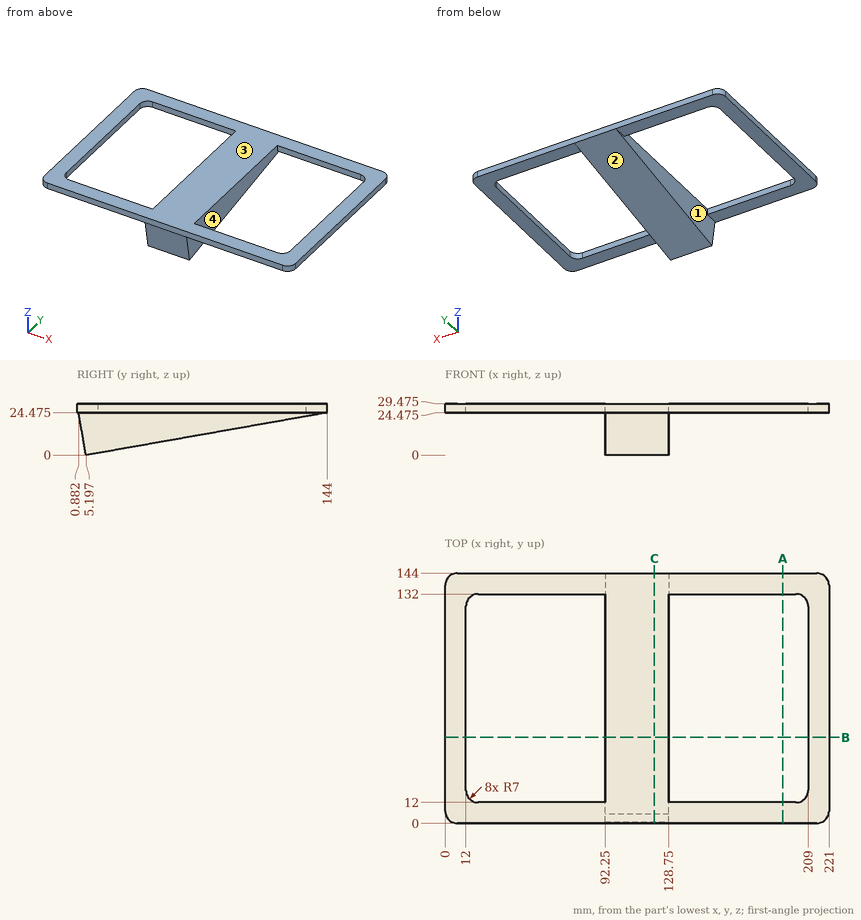
Part print with two shaded views. Sizes in mm from the minimum x, y, z corner. A direction names the side the tool comes from. Give positions to 0.01 mm unless a question says otherwise; leave off trailing zeros. Order: outer loops, then holes, each group sorted by start corner. A loop starts at its lowest first (then second) coordinate and runs counter-clockwise, first axis right, second up. Notation, with made-up numbers: M 59.5,35.25 L 114.5,35.25 A26 ccw 114.5,69.25 Z; hole C 73.25,40 d10. An arc over 180 degrees is marked long. Write item = value, one per line.
Q1. Two-plate mould, pull along X, no slides. Class the marked faces 3 and 4: pulls with the +X half, pulls with the -X half, needs draft (parallel to the pull), parting line crosses it, or undercut.
Derived:
face_3 = needs draft
face_4 = undercut
Q2. Cut at C-C, the plane x = 120.5. List the corners of the cut face in (y, z) (1 decimal), then the cut area to 3 significant figures.
Derived:
outline = M 0,24.5 L 0.9,24.5 L 5.2,0 L 144,24.5 L 144,29.5 L 0,29.5 Z
area = 2,470 mm2
Q3. Drill centre lines: line 1 (X direction, y = 23, z = 26.5); line 2 (X direction, y = 65.5, z = 20). Where is each one in solid material? Low to high. Write a range as [from, to].
Derived:
line_1 = [0, 12], [92.25, 128.75], [209, 221]
line_2 = [92.25, 128.75]
Q4. Flat gauge pins, fed straight in: pin 1 (9 mm diameter, centred on y = 59.5, z = 16.5, fed in from -X); pin 2 (5 mm diameter, centred on y = 78.5, z = 20, fed in from +X); pin 3 (8 mm diameter, centred on x = 117, z = 5.5, fed in from -Y). Where does each tip first touch, or does it go through?
Derived:
pin_1 = 92.25
pin_2 = 128.75
pin_3 = 3.52
Q5. Cut at B-B, the plane y = 49.5. Count the separate pieces of the cut face and the enclosed holes in it, then the cut area to 3 significant figures.
Derived:
separate_pieces = 3
enclosed_holes = 0
area = 911 mm2
Q6. Cut at A-A, the plane x = 194.5. List the corners of the cut face in (y, z) (1 decimal).
Derived:
outline = M 0,24.5 L 12,24.5 L 12,29.5 L 0,29.5 Z; M 132,24.5 L 144,24.5 L 144,29.5 L 132,29.5 Z
Q7. Tool access for the marked faces 1 and 2: list every direction of +Z, -Z, +X, -X, +Y, -Y with a clear straight run to the whole face (end or side of a thin tool).
Derived:
face_1 = -Z
face_2 = -Z, +X, -X, +Y
